from build123d import *

# Parameters (mm, degrees)
F1_DEPTH  = 4
F3_DEPTH  = 4
F4_W      = 10
F4_H      = 10
F5_DEPTH  = 24.7904
F7_DEPTH  = 10
F9_DEPTH  = 4
F4_H_2    = 3
F4_H_3    = 4
F11_DEPTH = 0.01


with BuildPart() as f1:
    # F0 (on Front) → F1 (new body)
    with BuildSketch(Plane.XZ):
        Polygon((239.7020892799, 112.8335457823), (-265.2979107201, 112.8335457823), (-265.2979107201, -137.1664542177), (239.7020892799, 97.8335457823), align=None)
    extrude(amount=F1_DEPTH)

    # F2 (on face) → F3 (cut)
    with BuildSketch(Plane.XZ.offset(4)):
        Polygon((211.2594902502, 97.8335457823), (189.459964633, 97.8335457823), (-257.2979107201, 97.8335457823), (-257.2979107201, -120.2080170455), (191.9194537148, 88.8337268004), align=None)
    extrude(amount=-F3_DEPTH, mode=Mode.SUBTRACT)

    # F4 (on face) → F5 (join)
    with BuildSketch(Plane.XY.offset(112.8335457823)):
        with Locations((234.7020892799, -2)):
            Rectangle(F4_W, F4_H)
    extrude(amount=-F5_DEPTH)

    # F6 (on face) → F7 (cut)
    with BuildSketch(Plane(origin=(229.7020892799, 0, 0), x_dir=(0, -1, 0), z_dir=(-1, 0, 0))):
        Polygon((7, 112.8335457823), (4, 93.1800804357), (0, 93.1800804357), (-3, 112.8335457823), (-3, 88.0431457823), (7, 88.0431457823), align=None)
    extrude(amount=-F7_DEPTH, mode=Mode.SUBTRACT)

    # F4 (on face) → F11 (join)
    with BuildSketch(Plane.XY.offset(112.8335457823)):
        with Locations((234.7020892799, 1.5)):
            Rectangle(F4_W, F4_H_2)
        with Locations((234.7020892799, -2)):
            Rectangle(F4_W, F4_H_3)
        with Locations((234.7020892799, -5.5)):
            Rectangle(F4_W, F4_H_2)
    extrude(amount=F11_DEPTH)


with BuildPart() as f9:
    # F8 (on face) → F9 (new body)
    with BuildSketch(Plane.XZ.offset(4)):
        Polygon((-265.2979107201, -137.1664542177), (241.7362299691, 93.1800804357), (229.7020892799, 93.1800804357), align=None)
    extrude(amount=-F9_DEPTH)


solid = f1.part
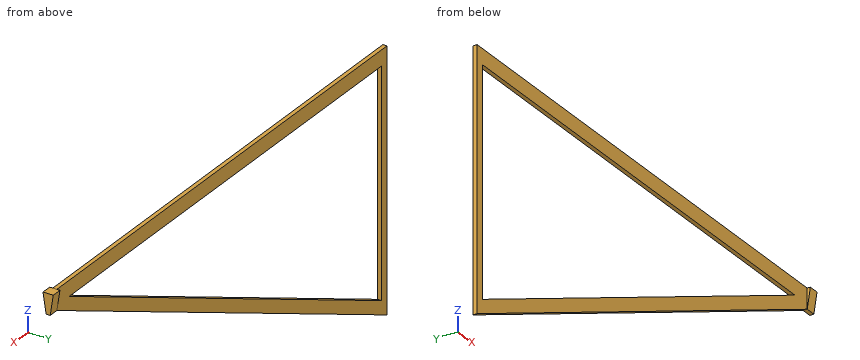
Can you work these out from the model? Positions are in its coordinate system, mm. Round coordinates to 2 decimals unless told otherwise and drop trailing zeros. Loops run counter-clockwise (first coordinate to the right, second up) from the corner with the lowest first, then second, coordinate; pieces in that order, holes last. Notation, with made-up numbers: (12, 63) - (70, 63) arc R33 cw to (70, 101) - close; hole circle Ø5 at (56, 5). An arc over 180 degrees is marked (long way). Write item = value, one per line. Start each with the question number.
(1) If we section it at C-C (z = -98.5): Please give me the cut outline in (x, y).
(2) For P1, Ø4.5, axis at x = 53.5, y = -2.5, coming from the +Z side; P2, Ø4, axis at y = -2.5, z = 64, coming from the +X side; P3, Ø3, axis at x = 0.5, y = -2.5, coming from the -Z side, each with a flat end and sliding along its axis, tell me the tip position at first contact or that it passes through.
(3) If we section it at B-B (x = 88): Please give me the cut outline in (y, z).
(4) If I drill on probe 1 along X at (y, z) = (0.5, 102); probe 2 along Z at (x, y) = (-195, -2.5); probe 3 along Y at (x, z) = (23.5, 99.5), over which ranges is the centre line in solid material (lowest first)? Write a range as [from, to].
Ans:
q1.outline = (-265.3, -4) - (-257.3, -4) - (-257.3, 0) - (-265.3, 0) - close; (-210.65, -4) - (-182.21, -4) - (-182.21, 0) - (-210.65, 0) - close
q2.P1 = 112.83
q2.P2 = 171.29
q2.P3 = -14.18
q3.outline = (-4, 27.24) - (0, 27.24) - (0, 40.48) - (-4, 40.48) - close; (-4, 97.83) - (0, 97.83) - (0, 112.83) - (-4, 112.83) - close
q4.probe_1 = [229.7, 239.7]
q4.probe_2 = [-104.45, -91.22], [97.83, 112.83]
q4.probe_3 = [-4, 0]
